from build123d import *

# Parameters (mm, degrees)
F1_DEPTH = 12.7
F3_DEPTH = 12.7
F5_DEPTH = 25.4
F7_DEPTH = 12.7


with BuildPart() as f1:
    # F0 (on Front) → F1 (new body)
    with BuildSketch(Plane.XZ):
        Polygon((-53.534672, 31.75), (-53.534672, 0), (3.615328, 0), (-9.084672, 31.75), align=None)
    extrude(amount=F1_DEPTH)

    # F2 (on Front) → F3 (join)
    with BuildSketch(Plane.XZ):
        Polygon((-53.729344, 31.75), (-53.729344, 0), (-21.979344, 0), (-34.679344, 31.75), align=None)
    extrude(amount=F3_DEPTH)

    # F4 (on Front) → F5 (join)
    with BuildSketch(Plane.XZ):
        Polygon((-53.729344, 31.75), (-53.729344, 0), (-21.979344, 0), (-34.679344, 31.75), align=None)
    extrude(amount=F5_DEPTH)

    # F6 (on face) → F7 (join)
    with BuildSketch(Plane(origin=(0, 0, 0), x_dir=(-1, 0, 0), z_dir=(0, 1, 0))):
        Polygon((21.979344, 0), (53.729344, 0), (53.729344, 31.75), (31.407008, 31.75), align=None)
    extrude(amount=F7_DEPTH)


solid = f1.part
CAD build for the part. Positions are in the model's coordinates, mm. A direction names the side the tool comes from. Round coordinates to 2 decimals unless told otherwise and drop trailing zeros. Order: outer loops, then holes, each group sorted by start corner. A loop starts at its lowest first (then second) coordinate and runs counter-clockwise, first axis right, second up. Notation, with made-up numbers: (62, -3.75) -> (68, -3.75) arc R16 ccw to (68, 2.25) -> close; hole circle Ø3 at (-40, -10.75). An arc over 180 degrees is marked (long way). Write item = value, one per line. Start each with the question number.
(1) Cut at C-C, the plane x = -24.5. List the corners of the cut face in (y, z), then the cut area to 3 significant figures.
(2) Cut at A-A, the plane z = 12. List the corners of the cut face in (x, y).
(3) Cut at B-B, the plane y = 9.5. List the corners of the cut face in (x, z), then the cut area to 3 significant figures.
(4) Pin check, flat tips, straight feed: P1, Ø9.5, axis at x = -24, z = 20.5, coming from the -Y side; P2, Ø2, axis at y = -3, z = 24, coming from the +X side; P3, Ø16, axis at x = -9, z = 18, coming from the +Y side. Stop position of each tip, or through.
(5) Which spindle directions (+Z, -Z, +X, -X, +Y, -Y) get a long thin tool onto all of the face, cutting with end or side? Do faces 1 (the flat face through (-14, 0, 16)), 2 (the flat face through (-37, -7, 31.75)), 3 (the flat face through (-16, -12.7, 16)). Say none if no direction does.
(6) Cut at D-D, the plane y = -14. List the corners of the cut face in (x, z).
(7) Probe line 1 (Y direction, x = -27.5, z = 30); line 2 (X direction, y = -17.5, z = 21.5); line 3 (X direction, y = -2, z = 25.5). List the from-to ranges inside material, lowest first. Write a range as [from, to].
Model answer:
q1.outline = (-25.4, 0) -> (12.7, 0) -> (12.7, 8.49) -> (0, 8.49) -> (0, 31.75) -> (-12.7, 31.75) -> (-12.7, 6.3) -> (-25.4, 6.3) -> close
q1.area = 591 mm2
q2.outline = (-53.73, -25.4) -> (-26.78, -25.4) -> (-26.78, -12.7) -> (-1.18, -12.7) -> (-1.18, 0) -> (-25.54, 0) -> (-25.54, 12.7) -> (-53.73, 12.7) -> close
q3.outline = (-53.73, 0) -> (-21.98, 0) -> (-31.41, 31.75) -> (-53.73, 31.75) -> close
q3.area = 858 mm2
q4.P1 = -12.7
q4.P2 = -5.58
q4.P3 = 0
q5.face_1 = +Z, +X, +Y
q5.face_2 = +Z, +X, -X, +Y, -Y
q5.face_3 = +Z, +X, -Y
q6.outline = (-53.73, 0) -> (-21.98, 0) -> (-34.68, 31.75) -> (-53.73, 31.75) -> close
q7.line_1 = [-12.7, 0]
q7.line_2 = [-53.73, -30.58]
q7.line_3 = [-53.73, -6.58]
